Could you check a few things on this model? Use its own coordinates, in mm. Give positions to 0.01 mm unless a question says otherwise; leave off trailing zeros. Order: outer loops, then holes, each group sorted by start corner. A loop starts at its lowest first (then second) coordinate and runs counter-clockwise, first axis right, second up. Notation, with made-up numbers: (43.5, 14) - (95.5, 14) arc R22 ccw to (95.5, 28) - close; hole circle Ø1 at (70, 25). An arc over 180 degrees is marked (long way). Put each result on its own line as item: value.
from build123d import *

# Parameters (mm, degrees)
BOSS_EXTRUDE1_DEPTH = 10
SKETCH2_R           = 1
SKETCH2_R_2         = 1.5
SKETCH2_W           = 33
SKETCH2_H           = 10
CUT_EXTRUDE2_DEPTH  = 15
SKETCH3_R           = 10
CUT_EXTRUDE3_DEPTH  = 5
CUT_EXTRUDE4_DEPTH  = 15
SKETCH5_W           = 30
SKETCH5_H           = 1
SKETCH5_W_2         = 1
SKETCH5_H_2         = 30
SKETCH5_H_3         = 15
CUT_EXTRUDE6_DEPTH  = 15
SKETCH6_R           = 0.5
CUT_EXTRUDE7_DEPTH  = 15


with BuildPart() as part:
    # Sketch1 → Boss-Extrude1 (new body)
    with BuildSketch(Plane(origin=(0, 0, 0), x_dir=(1, 0, 0), z_dir=(0, 1, 0))):
        with BuildLine():
            Line((-89.389143795, -90), (-89.389143795, 90))
            Line((-89.389143795, 90), (10.610856205, 90))
            ThreePointArc((10.610856205, 90), (54.533138364, 81.496268076), (92.107774725, 57.214031174))
            ThreePointArc((92.107774725, 57.214031174), (94.381847518, 53.920998768), (95.182620993, 50))
            Line((95.182620993, 50), (95.182620993, -50))
            ThreePointArc((95.182620993, -50), (94.381847518, -53.920998768), (92.107774725, -57.214031174))
            ThreePointArc((92.107774725, -57.214031174), (54.533138364, -81.496268076), (10.610856205, -90))
            Line((10.610856205, -90), (-89.389143795, -90))
        make_face()
    extrude(amount=BOSS_EXTRUDE1_DEPTH)

    # Sketch2 → Cut-Extrude2 (cut, symmetric)
    with BuildSketch(Plane(origin=(0, 10, 0), x_dir=(1, 0, 0), z_dir=(0, 1, 0))):
        with Locations(Location((65, 14.131573434, 0), (0, 0, 90))):
            Circle(SKETCH2_R)
        with Locations(Location((27.688972694, 9.173126615, 0), (0, 0, 90))):
            Circle(SKETCH2_R_2)
        with Locations(Location((14.053243942, 9.173126615, 0), (0, 0, 90))):
            Circle(SKETCH2_R_2)
        with Locations(Location((14.053243942, -9.173126615, 0), (0, 0, 90))):
            Circle(SKETCH2_R_2)
        with Locations(Location((27.688972694, -9.173126615, 0), (0, 0, 90))):
            Circle(SKETCH2_R_2)
        with Locations(Location((65, -14.131573434, 0), (0, 0, 90))):
            Circle(SKETCH2_R)
        with BuildLine():
            Line((-40.968894473, 86.42714575), (-40.968894473, 80.97285425))
            ThreePointArc((-40.968894473, 80.97285425), (-43.204350858, 78.737397865), (-45.439807243, 80.97285425))
            Line((-45.439807243, 80.97285425), (-45.439807243, 86.42714575))
            ThreePointArc((-45.439807243, 86.42714575), (-43.204350858, 88.662602135), (-40.968894473, 86.42714575))
        make_face()
        with BuildLine():
            Line((38.845478036, 11.594873944), (38.845478036, 4.405126056))
            ThreePointArc((38.845478036, 4.405126056), (36.366254627, 1.925902647), (33.887031217, 4.405126056))
            Line((33.887031217, 4.405126056), (33.887031217, 11.594873944))
            ThreePointArc((33.887031217, 11.594873944), (36.366254627, 14.074097353), (38.845478036, 11.594873944))
        make_face()
        with Locations((-64.401012641, 85)):
            Rectangle(SKETCH2_W, SKETCH2_H)
        with BuildLine():
            Line((38.845478036, -11.594873944), (38.845478036, -4.405126056))
            ThreePointArc((38.845478036, -4.405126056), (36.366254627, -1.925902647), (33.887031217, -4.405126056))
            Line((33.887031217, -4.405126056), (33.887031217, -11.594873944))
            ThreePointArc((33.887031217, -11.594873944), (36.366254627, -14.074097353), (38.845478036, -11.594873944))
        make_face()
        with BuildLine():
            Line((-40.968894473, -86.42714575), (-40.968894473, -80.97285425))
            ThreePointArc((-40.968894473, -80.97285425), (-43.204350858, -78.737397865), (-45.439807243, -80.97285425))
            Line((-45.439807243, -80.97285425), (-45.439807243, -86.42714575))
            ThreePointArc((-45.439807243, -86.42714575), (-43.204350858, -88.662602135), (-40.968894473, -86.42714575))
        make_face()
        with Locations((-64.401012641, -85)):
            Rectangle(SKETCH2_W, SKETCH2_H)
    extrude(amount=CUT_EXTRUDE2_DEPTH, both=True, mode=Mode.SUBTRACT)

    # Sketch3 → Cut-Extrude3 (cut, symmetric)
    with BuildSketch(Plane(origin=(0, 10, 0), x_dir=(1, 0, 0), z_dir=(0, 1, 0))):
        with Locations(Location((82.479810043, 0, 0), (0, 0, 270))):
            Circle(SKETCH3_R)
    extrude(amount=CUT_EXTRUDE3_DEPTH, both=True, mode=Mode.SUBTRACT)

    # Sketch4 → Cut-Extrude4 (cut, symmetric)
    with BuildSketch(Plane(origin=(0, 10, 0), x_dir=(1, 0, 0), z_dir=(0, 1, 0))):
        with BuildLine():
            Line((49.010294015, 4.462602137), (60.91056638, 4.462602137))
            ThreePointArc((60.91056638, 4.462602137), (65.373168517, 0), (60.91056638, -4.462602137))
            Line((60.91056638, -4.462602137), (49.010294015, -4.462602137))
            ThreePointArc((49.010294015, -4.462602137), (44.547691878, 0), (49.010294015, 4.462602137))
        make_face()
    extrude(amount=CUT_EXTRUDE4_DEPTH, both=True, mode=Mode.SUBTRACT)

    # Sketch5 → Cut-Extrude6 (cut, symmetric)
    with BuildSketch(Plane(origin=(0, 10, 0), x_dir=(1, 0, 0), z_dir=(0, 1, 0))):
        with Locations((-7.901012641, 88.5)):
            Rectangle(SKETCH5_W, SKETCH5_H)
        with Locations((-87.889143795, 40)):
            Rectangle(SKETCH5_W_2, SKETCH5_H_2)
        with Locations((93.682620993, 27.5)):
            Rectangle(SKETCH5_W_2, SKETCH5_H_3)
        with Locations((93.682620993, -27.5)):
            Rectangle(SKETCH5_W_2, SKETCH5_H_3)
        with Locations((-7.901012641, -88.5)):
            Rectangle(SKETCH5_W, SKETCH5_H)
        with Locations((-87.889143795, -40)):
            Rectangle(SKETCH5_W_2, SKETCH5_H_2)
    extrude(amount=CUT_EXTRUDE6_DEPTH, both=True, mode=Mode.SUBTRACT)

    # Sketch6 → Cut-Extrude7 (cut, symmetric)
    with BuildSketch(Plane(origin=(0, 5, 0), x_dir=(1, 0, 0), z_dir=(0, 1, 0))):
        with Locations(Location((82.244112685, 2.835581496, 0), (0, 0, 270))):
            Circle(SKETCH6_R)
        with Locations(Location((82.244112685, -5.164418504, 0), (0, 0, 270))):
            Circle(SKETCH6_R)
    extrude(amount=CUT_EXTRUDE7_DEPTH, both=True, mode=Mode.SUBTRACT)


solid = part.part
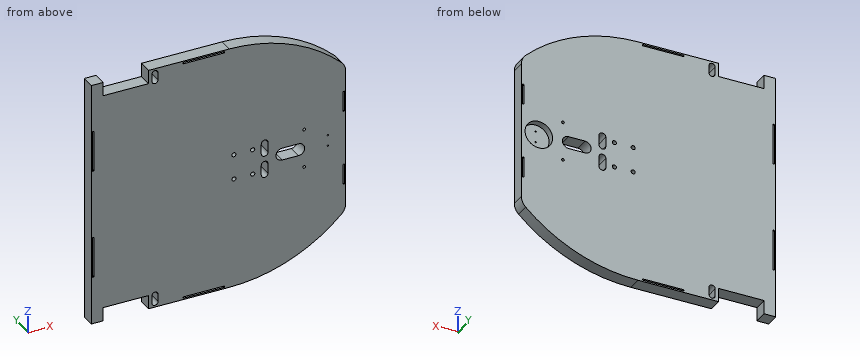
1) If I drill on line 1 (X direction, y = 8.7, z = 0); line 2 (Z direction, x = -7.5, y = 6.5); line 3 (X direction, y = 1, z = 37.5), over which ranges is the centre line in solid material (lowest first)? Write a range as [from, to].
Filled in:
line 1: x = [-89.39, 44.55], [65.37, 72.48], [92.48, 95.18]
line 2: z = [-90, -89], [-88, 88], [89, 90]
line 3: x = [-89.39, -88.39], [-87.39, 95.18]
2) Suppose I cut it at D-D, the plane x = 31.5. List the corners of the cut face in (y, z) for me.
Filled in:
outline: (0, -88.13) - (10, -88.13) - (10, 88.13) - (0, 88.13) - close
3) Suppose I cut it at C-C, the plane x = -51. List the corners of the cut face in (y, z) for me.
Filled in:
outline: (0, -80) - (10, -80) - (10, 80) - (0, 80) - close
4) I'm going to push flat-ended pins straight in: pin 1 (1.5 mm diameter, centred on x = 73, y = 5.5, fed in from -Z); pin 2 (0.8 mm diameter, centred on x = 94, y = 3, fed in from -Z); pin 3 (10 mm diameter, centred on x = 79.5, z = 2, fed in from +Y); pin 4 (2.5 mm diameter, centred on x = 27.69, z = 9.17, fed in from +Y). Where does each tip first touch, or does it pass through?
Filled in:
pin 1: stops at z = -72.57
pin 2: stops at z = -55.4
pin 3: stops at y = 5
pin 4: passes through
5) Suppose I cut it at A-A, the plane x = 54.5. List the corners of the cut face in (y, z) for me, and give its area (3 significant figures).
Filled in:
outline: (0, -81.51) - (10, -81.51) - (10, -4.46) - (0, -4.46) - close; (0, 4.46) - (10, 4.46) - (10, 81.51) - (0, 81.51) - close
area: 1,540 mm^2
6) Suppose I cut it at B-B, the plane y = 6.75. State how many separate pieces and enclosed holes the cut face has, and give its area (3 significant figures).
Filled in:
separate pieces: 1
enclosed holes: 18
area: 29,800 mm^2
